Work out the finished part from the listing and answer in its coordinate system (mm). A direction names the side the tool comes from. Give positions to 0.01 mm unless a question says otherwise; leave off trailing zeros. Loops run counter-clockwise (first coordinate to the right, second up) from the corner with the lowest first, then second, coordinate; pieces in that order, holes last.
from build123d import *

# Parameters (mm, degrees)
CROQUIS1_W              = 12.5
CROQUIS1_H              = 22.7
SALIENTE_EXTRUIR1_DEPTH = 23
SALIENTE_EXTRUIR2_DEPTH = 4
CROQUIS3_W              = 2.3
CROQUIS3_H              = 5
SALIENTE_EXTRUIR3_DEPTH = 6.25
CORTAR_EXTRUIR1_REACH   = 20.5
CROQUIS4_R              = 1
SALIENTE_EXTRUIR4_START = -4
CROQUIS5_W              = 4
CROQUIS5_H              = 5
SALIENTE_EXTRUIR4_DEPTH = 1.5
CROQUIS6_R              = 2.35
CROQUIS6_R_2            = 0.8
SALIENTE_EXTRUIR5_DEPTH = 2.4
SKETCH1_W               = 4.514706964
SKETCH1_H               = 2.103718672
CUT_EXTRUDE2_DEPTH      = 5


with BuildPart() as part:
    # Croquis1 → Saliente-Extruir1 (new body)
    with BuildSketch(Plane.XY):
        Rectangle(CROQUIS1_W, CROQUIS1_H)
    extrude(amount=SALIENTE_EXTRUIR1_DEPTH)

    # Croquis2 → Saliente-Extruir2 (add)
    with BuildSketch(Plane.XY.offset(23)):
        with BuildLine():
            Line((2.9, 0.265128397), (2.9, -0.634871603))
            ThreePointArc((2.9, -0.634871603), (0, -11.35), (-2.9, -0.634871603))
            Line((-2.9, -0.634871603), (-2.9, 0.265128397))
            ThreePointArc((-2.9, 0.265128397), (0, 3.165128397), (2.9, 0.265128397))
        make_face()
    extrude(amount=SALIENTE_EXTRUIR2_DEPTH)

    # Croquis3 → Saliente-Extruir3 (add, symmetric)
    with BuildSketch(Plane(origin=(0, 0, 0), x_dir=(0, 0, -1), z_dir=(1, 0, 0))):
        with Locations((-17.35, 13.85)):
            Rectangle(CROQUIS3_W, CROQUIS3_H)
        with Locations((-17.35, -13.85)):
            Rectangle(CROQUIS3_W, CROQUIS3_H)
    extrude(amount=SALIENTE_EXTRUIR3_DEPTH, both=True)

    # Croquis4 → Cortar-Extruir1 (cut, up to next)
    with BuildSketch(Plane.XY.offset(18.5), mode=Mode.PRIVATE) as cortar_extruir1_sk1:
        with Locations((0, 13.85)):
            Circle(CROQUIS4_R)
    cortar_extruir1_tool1 = extrude(cortar_extruir1_sk1.sketch, amount=-CORTAR_EXTRUIR1_REACH, mode=Mode.PRIVATE) & part.part
    add(cortar_extruir1_tool1.solids().sort_by_distance((0, 13.85, 18.5))[0], mode=Mode.SUBTRACT)
    # Croquis4 → Cortar-Extruir1 (cut, up to next)
    with BuildSketch(Plane.XY.offset(18.5), mode=Mode.PRIVATE) as cortar_extruir1_sk2:
        with Locations((0, -13.85)):
            Circle(CROQUIS4_R)
    cortar_extruir1_tool2 = extrude(cortar_extruir1_sk2.sketch, amount=-CORTAR_EXTRUIR1_REACH, mode=Mode.PRIVATE) & part.part
    add(cortar_extruir1_tool2.solids().sort_by_distance((0, -13.85, 18.5))[0], mode=Mode.SUBTRACT)

    # Croquis5 → Saliente-Extruir4 (add)
    with BuildSketch(Plane(origin=(0, 0, 0), x_dir=(-1, 0, 0), z_dir=(0, 0, -1)).offset(SALIENTE_EXTRUIR4_START)):
        with Locations((0, -13.85)):
            Rectangle(CROQUIS5_W, CROQUIS5_H)
    extrude(amount=-SALIENTE_EXTRUIR4_DEPTH)

    # Croquis6 → Saliente-Extruir5 (add)
    with BuildSketch(Plane.XY.offset(27)):
        with Locations((0, -5.6)):
            Circle(CROQUIS6_R)
        with Locations((0, -5.6)):
            Circle(CROQUIS6_R_2, mode=Mode.SUBTRACT)
    extrude(amount=SALIENTE_EXTRUIR5_DEPTH)

    # Sketch1 → Cut-Extrude2 (cut)
    with BuildSketch(Plane.XZ.offset(16.35)):
        with Locations((0, 4.75)):
            Rectangle(SKETCH1_W, SKETCH1_H)
        with BuildLine():
            ThreePointArc((-0.625, 4.335421901), (-2, 4.75), (-0.625, 5.164578099))
            ThreePointArc((-0.625, 5.164578099), (0, 5.5), (0.625, 5.164578099))
            ThreePointArc((0.625, 5.164578099), (2, 4.75), (0.625, 4.335421901))
            ThreePointArc((0.625, 4.335421901), (0, 4), (-0.625, 4.335421901))
        make_face(mode=Mode.SUBTRACT)
    extrude(amount=-CUT_EXTRUDE2_DEPTH, mode=Mode.SUBTRACT)


solid = part.part
Item 1: Find section D-D, the plane x = -4.75. Write down the section's boundary in (y, z), plus the area to 3 significant figures.
Item 2: Find section A-A, the plane y = 13.85. Write down the section's boundary in (x, z), plus the area to 4 significant figures.
Item 3: Find section B-B, the plane z = 4.75. Write down the section's boundary in (x, y).
Item 4: Consider line 1 (Y direction, x = 0, z = 17.5); line 2 (Y direction, x = 0, z = 27.8); line 3 (Y direction, x = 2.5, z = 5.25). Determine where each line is inside the solid, lowest interval first.
Item 5: Flat-ended cylindrical pins translate along their axes: pin 1 Ø1.5 at (x, z) = (4, 13) entering from +Y; pin 2 Ø6 at (x, y) = (-0.5, 8.5) entering from +Z; pin 3 Ø2.5 at (x, y) = (1, 14) entering from -Z. Find the tip coordinate at first contact, or state that the pin passes through.
Item 6: For faces 1 (the face through (-0.509, -7.894, 28.183)), 2 (the face through (2.9, 0, 25)), 3 (the face through (0, -15, 16.2)), 4 (the face through (0, -15, 18.5)), 5 (the face through (-2.9, 0, 25)), determine the directions among +Z, -Z, +X, -X, +Y, -Y from which every point of the face is accessible in a straight line to the end or side of a thin tool.
Item 7: Determine the mould class of faces 6 (the face through (-0.13, -12.86, 17.37)), 7 (the face through (0, 11.35, 21)), 8 (the face through (-0.217, 12.874, 17.366)), 9 (the face through (0, -16.35, 5)) for opening direction Y: released by +Y, released by -Y, zero draft, split by the parting line, or undercut.
Item 8: Find section C-C, the plane y = 2. Write down the section's boundary in (x, z).
Ans:
1. outline: (-16.35, 16.2) - (-11.35, 16.2) - (-11.35, 0) - (11.35, 0) - (11.35, 16.2) - (16.35, 16.2) - (16.35, 18.5) - (11.35, 18.5) - (11.35, 23) - (-2.36, 23) - (-2.36, 27) - (-8.84, 27) - (-8.84, 23) - (-11.35, 23) - (-11.35, 18.5) - (-16.35, 18.5) - close
1. area: 571 mm2
2. outline: (-6.25, 16.2) - (-1, 16.2) - (-1, 18.5) - (-6.25, 18.5) - close; (1, 16.2) - (6.25, 16.2) - (6.25, 18.5) - (1, 18.5) - close
2. area: 24.15 mm2
3. outline: (-6.25, -11.35) - (-2, -11.35) - (-2, -16.35) - (2, -16.35) - (2, -11.35) - (6.25, -11.35) - (6.25, 11.35) - (-6.25, 11.35) - close
4. line 1: y = -16.35 to -14.85, -12.85 to 12.85, 14.85 to 16.35
4. line 2: y = -7.95 to -6.4, -4.8 to -3.25
4. line 3: y = -11.35 to 11.35
5. pin 1: stops at y = 11.35
5. pin 2: stops at z = 23
5. pin 3: stops at z = 16.2
6. face 1: +Z
6. face 2: +Z, +X, +Y
6. face 3: +X, -X, -Y
6. face 4: +Z, +X, -X, -Y
6. face 5: +Z, -X, +Y
7. face 6: undercut
7. face 7: released by +Y
7. face 8: undercut
7. face 9: released by -Y
8. outline: (-6.25, 0) - (6.25, 0) - (6.25, 23) - (2.32, 23) - (2.32, 27) - (-2.32, 27) - (-2.32, 23) - (-6.25, 23) - close
